from build123d import *

# Parameters (mm, degrees)
EXTRUDE_1_DEPTH          = 3
CUT_EXTRUDE_1_DEPTH      = 42
CUT_EXTRUDE_1_DEPTH_BACK = 10
SKETCH_2_R               = 1.4
SKETCH_3_R               = 2.5
CUT_EXTRUDE_2_DEPTH      = 1.8
SKETCH_7_R               = 6
EXTRUDE_4_DEPTH          = 14
BUTTON_LEFT_NUT_DEPTH    = 5
UP_LEFT_NUT_DEPTH        = 5
UP_RIGHT_NUT_DEPTH       = 5
BUTTON_RIGHT_NUT_DEPTH   = 5
SKETCH_13_R              = 3.25
CUT_EXTRUDE_7_DEPTH      = 13
SKETCH_15_R              = 3.25
CUT_EXTRUDE_8_DEPTH      = 13
SKETCH_16_R              = 3.25
CUT_EXTRUDE_9_DEPTH      = 13
SKETCH_17_R              = 3.25
CUT_EXTRUDE_10_DEPTH     = 13


with BuildPart() as part:
    # 草图1 → 凸台-拉伸1 (new body)
    with BuildSketch(Plane.XY):
        with BuildLine():
            Line((-72.574116531, 45.487390308), (77.425883469, 45.487390308))
            ThreePointArc((77.425883469, 45.487390308), (84.496951281, 42.558458119), (87.425883469, 35.487390308))
            Line((87.425883469, 35.487390308), (87.425883469, -34.512609692))
            ThreePointArc((87.425883469, -34.512609692), (84.496951281, -41.583677504), (77.425883469, -44.512609692))
            Line((77.425883469, -44.512609692), (-72.574116531, -44.512609692))
            ThreePointArc((-72.574116531, -44.512609692), (-79.645184343, -41.583677504), (-82.574116531, -34.512609692))
            Line((-82.574116531, -34.512609692), (-82.574116531, 35.487390308))
            ThreePointArc((-82.574116531, 35.487390308), (-79.645184343, 42.558458119), (-72.574116531, 45.487390308))
        make_face()
    extrude(amount=EXTRUDE_1_DEPTH)

    # 草图2 → 切除-拉伸1 (cut, two sides: drawn at the far end of the back side and taken through both)
    with BuildSketch(Plane.XY.offset(3).offset(-CUT_EXTRUDE_1_DEPTH_BACK)):
        with Locations((-32.574116531, 12.987390308)):
            Circle(SKETCH_2_R)
        with Locations((-32.574116531, -12.012609692)):
            Circle(SKETCH_2_R)
        with Locations((37.425883469, 12.987390308)):
            Circle(SKETCH_2_R)
        with Locations((37.425883469, -12.012609692)):
            Circle(SKETCH_2_R)
        with BuildLine():
            Line((-60.749662301, -44.512609692), (60.437772164, -44.512609692))
            ThreePointArc((60.437772164, -44.512609692), (32.253211404, -33.835942142), (2.425883469, -29.512609692))
            ThreePointArc((2.425883469, -29.512609692), (-29.983273004, -33.55318593), (-60.749662301, -44.512609692))
        make_face()
        with BuildLine():
            Line((-62.574116531, 45.487390308), (67.425883469, 45.487390308))
            ThreePointArc((67.425883469, 45.487390308), (35.747267057, 34.428061428), (2.425883469, 30.487390308))
            ThreePointArc((2.425883469, 30.487390308), (-30.918540876, 34.328218147), (-62.574116531, 45.487390308))
        make_face()
        with BuildLine():
            Line((87.425883469, 20.487390308), (87.425883469, -19.512609692))
            ThreePointArc((87.425883469, -19.512609692), (76.286181126, -12.242386449), (72.425883469, 0.487390308))
            ThreePointArc((72.425883469, 0.487390308), (76.286181126, 13.217167065), (87.425883469, 20.487390308))
        make_face()
        with BuildLine():
            Line((-82.574116531, 20.487390308), (-82.574116531, -19.512609692))
            ThreePointArc((-82.574116531, -19.512609692), (-71.434414188, -12.242386449), (-67.574116531, 0.487390308))
            ThreePointArc((-67.574116531, 0.487390308), (-71.434414188, 13.217167065), (-82.574116531, 20.487390308))
        make_face()
        with BuildLine():
            Line((-17.574116531, 20), (22.425883469, 20))
            ThreePointArc((22.425883469, 20), (27.425883469, 15), (22.425883469, 10))
            Line((22.425883469, 10), (-17.574116531, 10))
            ThreePointArc((-17.574116531, 10), (-22.574116531, 15), (-17.574116531, 20))
        make_face()
        with BuildLine():
            Line((-17.079364826, 5), (22.920635174, 5))
            ThreePointArc((22.920635174, 5), (27.920635174, 0), (22.920635174, -5))
            Line((22.920635174, -5), (-17.079364826, -5))
            ThreePointArc((-17.079364826, -5), (-22.079364826, 0), (-17.079364826, 5))
        make_face()
        with BuildLine():
            Line((-17.079364826, -10), (22.920635174, -10))
            ThreePointArc((22.920635174, -10), (27.920635174, -15), (22.920635174, -20))
            Line((22.920635174, -20), (-17.079364826, -20))
            ThreePointArc((-17.079364826, -20), (-22.079364826, -15), (-17.079364826, -10))
        make_face()
    extrude(amount=CUT_EXTRUDE_1_DEPTH + CUT_EXTRUDE_1_DEPTH_BACK, mode=Mode.SUBTRACT)

    # 草图3 → 切除-拉伸2 (cut)
    with BuildSketch(Plane.XY.offset(3)):
        with Locations((-32.574116531, 12.987390308)):
            Circle(SKETCH_3_R)
        with Locations((37.425883469, 12.987390308)):
            Circle(SKETCH_3_R)
        with Locations((37.425883469, -12.012609692)):
            Circle(SKETCH_3_R)
        with Locations((-32.574116531, -12.012609692)):
            Circle(SKETCH_3_R)
    extrude(amount=-CUT_EXTRUDE_2_DEPTH, mode=Mode.SUBTRACT)

    # 草图7 → 凸台-拉伸4 (add)
    with BuildSketch(Plane.XY.offset(3)):
        with Locations(Location((-74.574116531, 37.487390308, 0), (0, 0, 180))):
            Circle(SKETCH_7_R)
        with Locations(Location((-74.574116531, -36.512609692, 0), (0, 0, 180))):
            Circle(SKETCH_7_R)
        with Locations(Location((79.425883469, 37.487390308, 0), (0, 0, 180))):
            Circle(SKETCH_7_R)
        with Locations(Location((79.425883469, -36.512609692, 0), (0, 0, 180))):
            Circle(SKETCH_7_R)
    extrude(amount=EXTRUDE_4_DEPTH)

    # 草图9 → button left nut (cut)
    with BuildSketch(Plane.XY.offset(17)):
        Polygon((-69.81097595, -39.262610189), (-69.81097595, -33.762609196), (-74.574116531, -31.0126087), (-79.337257112, -33.762609196), (-79.337257112, -39.262610189), (-74.574116531, -42.012610685), align=None)
    extrude(amount=-BUTTON_LEFT_NUT_DEPTH, mode=Mode.SUBTRACT)

    # 草图10 → up left nut (cut)
    with BuildSketch(Plane.XY.offset(17)):
        Polygon((-72.909327157, 32.245398669), (-69.202023918, 36.308144378), (-70.866813292, 41.550136017), (-76.238905905, 42.729381946), (-79.946209143, 38.666636237), (-78.28141977, 33.424644598), align=None)
    extrude(amount=-UP_LEFT_NUT_DEPTH, mode=Mode.SUBTRACT)

    # 草图11 → up right nut (cut)
    with BuildSketch(Plane.XY.offset(17)):
        Polygon((80.859330276, 32.177472205), (84.741130841, 36.073832606), (83.307684034, 41.383750708), (77.992436662, 42.79730841), (74.110636097, 38.900948009), (75.544082904, 33.591029907), align=None)
    extrude(amount=-UP_RIGHT_NUT_DEPTH, mode=Mode.SUBTRACT)

    # 草图12 → button right nut (cut)
    with BuildSketch(Plane.XY.offset(17)):
        Polygon((83.536634722, -40.166610806), (84.645716885, -34.779595236), (80.534965632, -31.125594122), (75.315132216, -32.858608579), (74.206050053, -38.245624149), (78.316801306, -41.899625263), align=None)
    extrude(amount=-BUTTON_RIGHT_NUT_DEPTH, mode=Mode.SUBTRACT)

    # 草图13 → 切除-拉伸7 (cut)
    with BuildSketch(Plane.XY.offset(17)):
        with Locations((-74.574116531, -36.512609692)):
            Circle(SKETCH_13_R)
    extrude(amount=-CUT_EXTRUDE_7_DEPTH, mode=Mode.SUBTRACT)

    # 草图15 → 切除-拉伸8 (cut)
    with BuildSketch(Plane.XY.offset(17)):
        with Locations((-74.574116531, 37.487390308)):
            Circle(SKETCH_15_R)
    extrude(amount=-CUT_EXTRUDE_8_DEPTH, mode=Mode.SUBTRACT)

    # 草图16 → 切除-拉伸9 (cut)
    with BuildSketch(Plane.XY.offset(17)):
        with Locations((79.425883469, 37.487390308)):
            Circle(SKETCH_16_R)
    extrude(amount=-CUT_EXTRUDE_9_DEPTH, mode=Mode.SUBTRACT)

    # 草图17 → 切除-拉伸10 (cut)
    with BuildSketch(Plane.XY.offset(17)):
        with Locations((79.425883469, -36.512609692)):
            Circle(SKETCH_17_R)
    extrude(amount=-CUT_EXTRUDE_10_DEPTH, mode=Mode.SUBTRACT)


solid = part.part
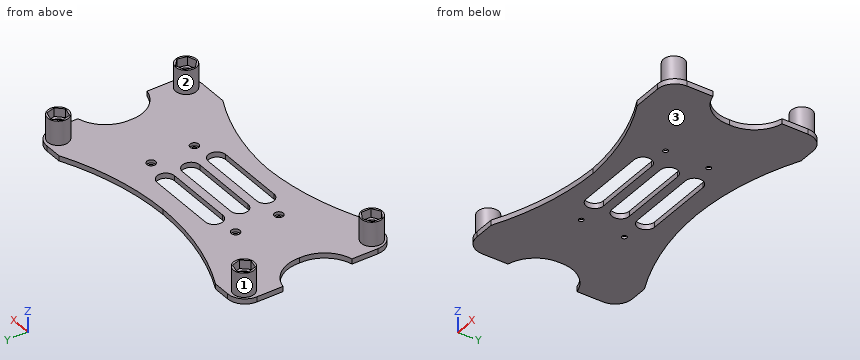
Could you check a few things on this model? Use its own coordinates, in mm. Face numbers are marked on the shaded views. Give positions to 0.01 mm unless a question says otherwise; leave off trailing zeros. Order: outer loops, then holes, each group sorted by start corner. A loop starts at its lowest first (then second) coordinate and runs counter-clockwise, first axis right, second up.
Item 1: I need wall thicknesses on line 1 (X direction, y = 35.5, z = 12.5); line 2 (Y direction, x = -3, z = 1.75); line 3 (Z direction, x = 32, y = 7.5). Which ranges of each line are inside material? Lowest first, please.
Item 2: If we mould it in two halves opening along X, with no side actions, what happens to the marked faces 1, 2 and 3? For each: pulls with the +X half, pulls with the -X half, needs draft (parallel to the pull), parting line crosses it, or undercut.
Item 3: I'm going to push flat-ended pins straight in: pin 1 (5 mm diameter, centred on x = -76, y = 38.5, fed in from +Z); pin 2 (3.5 mm diameter, centred on x = 7.5, z = 2, fed in from +Y); pin 3 (5 mm diameter, centred on x = 80, y = 37.5, fed in from +Z). Where does each tip first touch, or does it pass through?
Item 4: If we section it at B-B, the plane x = 15: Write out the boundary of the cut face in (y, z), plus the area to 3 significant figures.
Item 5: If we section it at C-C, the plane y = -17: Write out the boundary of the cut face in (x, z).
Item 6: If we section it at A-A, the plane z = 14: Write out the boundary of the cut face in (x, y), plus the area to 3 significant figures.
Values:
1. line 1: x = -80.24 to -78.94, -69.94 to -68.91, 73.76 to 75.03, 84.17 to 85.09
1. line 2: y = -29.69 to -20, -10 to -5, 5 to 10, 20 to 30.6
1. line 3: z = 0 to 3
2. face 1: undercut
2. face 2: undercut
2. face 3: needs draft
3. pin 1: stops at z = 12
3. pin 2: stops at y = 30.7
3. pin 3: stops at z = 4
4. outline: (-30.53, 0) - (-20, 0) - (-20, 3) - (-30.53, 3) - close; (-10, 0) - (-5, 0) - (-5, 3) - (-10, 3) - close; (5, 0) - (10, 0) - (10, 3) - (5, 3) - close; (20, 0) - (31.11, 0) - (31.11, 3) - (20, 3) - close
4. area: 94.9 mm2
5. outline: (-76.58, 0) - (-21.66, 0) - (-21.66, 3) - (-76.58, 3) - close; (27.5, 0) - (81.43, 0) - (81.43, 3) - (27.5, 3) - close
6. outline: circle Ø12 at (-74.57, -36.51); circle Ø12 at (-74.57, 37.49); circle Ø12 at (79.43, -36.51); circle Ø12 at (79.43, 37.49); hole (-79.95, 38.67) - (-78.28, 33.42) - (-72.91, 32.25) - (-69.2, 36.31) - (-70.87, 41.55) - (-76.24, 42.73) - close; hole (-79.34, -39.26) - (-74.57, -42.01) - (-69.81, -39.26) - (-69.81, -33.76) - (-74.57, -31.01) - (-79.34, -33.76) - close; hole (74.11, 38.9) - (75.54, 33.59) - (80.86, 32.18) - (84.74, 36.07) - (83.31, 41.38) - (77.99, 42.8) - close; hole (74.21, -38.25) - (78.32, -41.9) - (83.54, -40.17) - (84.65, -34.78) - (80.53, -31.13) - (75.32, -32.86) - close
6. area: 138 mm2
